Geometry: final body of the model. Coordinates: model frame, mm. Give positions to 0.01 mm unless a question says otherwise; leave off trailing zeros. Write each loop counter-clockwise with the first axis right and the second up, starting at its lowest first coordinate (ties: lowest second). Pieces come first, ordered by that corner, then holes. Notation, with made-up numbers: (15, 6) - (68, 6) arc R31 ccw to (68, 34) - close; hole circle Ø2 at (83, 39). An arc over 180 degrees is marked (long way). One line per question, with ' | ' between items. Start each with the question number.
```python
from build123d import *

# Parameters (mm, degrees)
F1_R     = 2.1
F2_DEPTH = 20


# Not quite as in the source:
# - ends of sketch curves that miss each other by under 0.0002 mm in the source are joined


with BuildPart() as f2:
    # F1 (on Top) → F2 (new body)
    with BuildSketch(Plane.XY):
        with BuildLine():
            Line((112.4458007812, 59.6080856323), (109.4554236891, 59.6080856323))
            Line((109.4554236891, 59.6080856323), (109.4554236891, 0))
            Line((109.4554236891, 0), (112.4458007812, 0))
            ThreePointArc((112.4458007812, 0), (117.7491016401, 2.1966991411), (119.9458007812, 7.5))
            add(Edge.make_bspline(
                [(119.9458007812, 52.1080865864), (119.9458007812, 37.238724391), (119.9458007812, 22.3693621955), (119.9458007812, 7.5)],
                knots=[0, 0, 0, 0, 1, 1, 1, 1], degree=3))
            ThreePointArc((119.9458007812, 52.1080865864), (117.7491016401, 57.4113864912), (112.4458007812, 59.6080856323))
        make_face()
        with Locations((114.4458007813, 6.9999980927)):
            Circle(F1_R, mode=Mode.SUBTRACT)
        with Locations((114.4458007813, 29.9999995232)):
            Circle(F1_R, mode=Mode.SUBTRACT)
        with Locations((114.4458007813, 52.9999995232)):
            Circle(F1_R, mode=Mode.SUBTRACT)
    extrude(amount=F2_DEPTH)


solid = f2.part
```
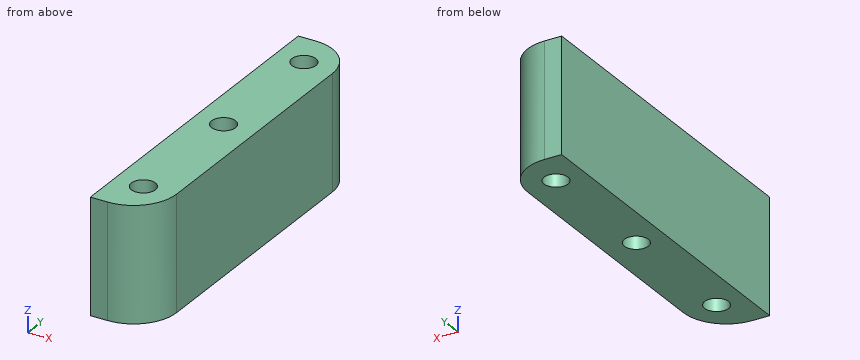
1) Line query: L1, parallel to Y at x = 113, z = 5.5; L2, parallel to Y at x = 113.75, z = 6; L3, parallel to X at y = 30, z = 14.75. Output: solid intervals per line, ascending.
2) Section A-A, the plane x = 113.75. Output: boundary loops of the cut face in (y, z).
3) Section C-C, the plane z = 8.75. Give the number of separate pieces and of enclosed holes in the cut face, plus the area to 3 significant figures.
4) Section B-B, the plane y = 53. Output: boundary loops of the cut face in (x, z), plus the area to 3 significant figures.
Answer key:
1) L1: 0.02 to 5.48, 8.52 to 28.48, 31.52 to 51.48, 54.52 to 59.59 | L2: 0.11 to 5.02, 8.98 to 28.02, 31.98 to 51.02, 54.98 to 59.49 | L3: 109.46 to 112.35, 116.55 to 119.95
2) outline: (0.11, 0) - (5.02, 0) - (5.02, 20) - (0.11, 20) - close; (8.98, 0) - (28.02, 0) - (28.02, 20) - (8.98, 20) - close; (31.98, 0) - (51.02, 0) - (51.02, 20) - (31.98, 20) - close; (54.98, 0) - (59.49, 0) - (59.49, 20) - (54.98, 20) - close
3) separate pieces: 1 | enclosed holes: 3 | area: 560 mm^2
4) outline: (109.46, 0) - (112.35, 0) - (112.35, 20) - (109.46, 20) - close; (116.55, 0) - (119.89, 0) - (119.89, 20) - (116.55, 20) - close | area: 125 mm^2
